from build123d import *

# Parameters (mm, degrees)
ESQUISSE1_W        = 30
ESQUISSE1_H        = 5
ESQUISSE1_R        = 1.346150104
BOSS_EXTRU_1_DEPTH = 3


with BuildPart() as part:
    # Esquisse1 → Boss.-Extru.1 (new body)
    with BuildSketch(Plane.XY):
        with Locations((15, 2.5)):
            Rectangle(ESQUISSE1_W, ESQUISSE1_H)
        with Locations((2.5, 2.5)):
            Circle(ESQUISSE1_R, mode=Mode.SUBTRACT)
        with Locations((27.5, 2.5)):
            Circle(ESQUISSE1_R, mode=Mode.SUBTRACT)
    extrude(amount=BOSS_EXTRU_1_DEPTH)


solid = part.part
The listing builds one solid part. Answer for the finished solid, in the listing's coordinates (mm). Coordinates: 2 decimals unless noted, no trailing zeros. Loops run counter-clockwise (first coordinate to the right, second up) from the corner with the lowest first, then second, coordinate; pieces in that order, holes last. Notation, with made-up numbers: M -21,47.5 L 20,47.5 A10 ccw 20,65.5 Z; hole C 85,-10.75 d1. An arc over 180 degrees is marked long. Answer in a Markdown table with one row per item.
1) Find section A-A (x = 2.5). Determine the outline of the cut face in (y, z), then the cut area to 3 significant figures.
Answers below:
| item | result |
|---|---|
| outline | M 0,0 L 1.15,0 L 1.15,3 L 0,3 Z; M 3.85,0 L 5,0 L 5,3 L 3.85,3 Z |
| area | 6.92 mm^2 |
2) Find section C-C (z = 1.2). Determine the outline of the cut face in (x, y), then the cut area to 3 significant figures.
Answers below:
| item | result |
|---|---|
| outline | M 0,0 L 30,0 L 30,5 L 0,5 Z; hole C 2.5,2.5 d2.69; hole C 27.5,2.5 d2.69 |
| area | 139 mm^2 |
3) Find the intervals of material crossed by probe 1 along Y at (x, z) = (2.5, 2.1); probe 2 along X at (y, z) = (1.55, 1.3); probe 3 along X at (y, z) = (1.7, 1.9), in increasing order.
Answers below:
| item | result |
|---|---|
| probe 1 | 0 to 1.15, 3.85 to 5 |
| probe 2 | 0 to 1.55, 3.45 to 26.55, 28.45 to 30 |
| probe 3 | 0 to 1.42, 3.58 to 26.42, 28.58 to 30 |
4) Determine the mould class of faces 1 (the flat face through (15, 5, 1)), 2 (the flat face through (0, 2, 1)), 3 (the cylindrical face through (2.325, 3.835, 1.479)) for opening direction X: released by +X, released by -X, zero draft, split by the parting line, or undercut.
Answers below:
| item | result |
|---|---|
| face 1 | zero draft |
| face 2 | released by -X |
| face 3 | undercut |
5) Find section B-B (y = 2.5). Determine the outline of the cut face in (x, z).
Answers below:
| item | result |
|---|---|
| outline | M 0,0 L 1.15,0 L 1.15,3 L 0,3 Z; M 3.85,0 L 26.15,0 L 26.15,3 L 3.85,3 Z; M 28.85,0 L 30,0 L 30,3 L 28.85,3 Z |
